Build history of the part. All positions in model axes, mm. Face numbers are marked on the shaded views. A direction names the side the tool comes from. Coordinates: 2 decimals unless noted, no trailing zeros. Loops run counter-clockwise (first coordinate to the right, second up) from the corner with the lowest first, then second, coordinate; pieces in that order, holes last.
(1) Slice it at A-A (z = 0). Give the cut face in (x, y) (3 decimals), and give its area (3 significant figures).
(2) Slice it at C-C (y = 9.25). Give the cut face in (x, z) (3 decimals).
(3) Two-plate mould, pull along X, no slides. Class the marked faces 3, 4 and 5: pulls with the +X half, pulls with the -X half, needs draft (parallel to the pull), parting line crosses it, or undercut.
(4) Wall check: L1, parallel to X at y = 11.75, z = 0 (3 decimals); L2, parallel to Y at x = 15.5, z = -11; L3, parallel to Z at x = 3, y = 4.25. Give the ranges that are in metal, low to high.
(5) Tool access for the marked faces 1 and 2: list every direction of +Z, -Z, +X, -X, +Y, -Y with a clear straight run to the whole face (end or side of a thin tool).
(6) Flat gauge pins, fed straight in: P1, Ø10, axis at y = 8, z = -2.5, coming from the -X side; P2, Ø1, axis at y = 17, z = -20, coming from the -X side; P3, Ø6, axis at x = -26.5, y = 11.5, coming from the +Z side; P4, Ø11.5, axis at x = 0, z = 0, coming from the -Y side. Where does each tip first touch, or does it go through?
(7) Slice it at B-B (x = 0). Give the cut face in (y, z) (3 decimals).
from build123d import *

# Parameters (mm, degrees)
SKETCH1_R           = 38.1
SKETCH1_R_2         = 9.525
BOSS_EXTRUDE1_DEPTH = 19.05
CHAMFER1_SIZE       = 2.54
SKETCH3_R           = 25.4
CUT_EXTRUDE2_DEPTH  = 6.35


with BuildPart() as part:
    # Sketch1 → Boss-Extrude1 (new body)
    with BuildSketch(Plane(origin=(0, 0, 0), x_dir=(1, 0, 0), z_dir=(0, 1, 0))):
        with Locations(Location((0, 0, 0), (0, 0, 90))):
            Circle(SKETCH1_R)
        with Locations(Location((0, 0, 0), (0, 0, 90))):
            Circle(SKETCH1_R_2, mode=Mode.SUBTRACT)
    extrude(amount=BOSS_EXTRUDE1_DEPTH)

    # Chamfer1
    chamfer1_edges = [part.edges().sort_by_distance(p)[0] for p in [
        (0, 0, 38.1),
        (0, 19.05, 38.1),
    ]]
    chamfer(chamfer1_edges, length=CHAMFER1_SIZE)

    # Sketch3 → Cut-Extrude2 (cut)
    with BuildSketch(Plane(origin=(0, 0, 0), x_dir=(-1, 0, 0), z_dir=(0, -1, 0))):
        with Locations(Location((0, 0, 0), (0, 0, 90))):
            Circle(SKETCH3_R)
    extrude(amount=-CUT_EXTRUDE2_DEPTH, mode=Mode.SUBTRACT)


solid = part.part
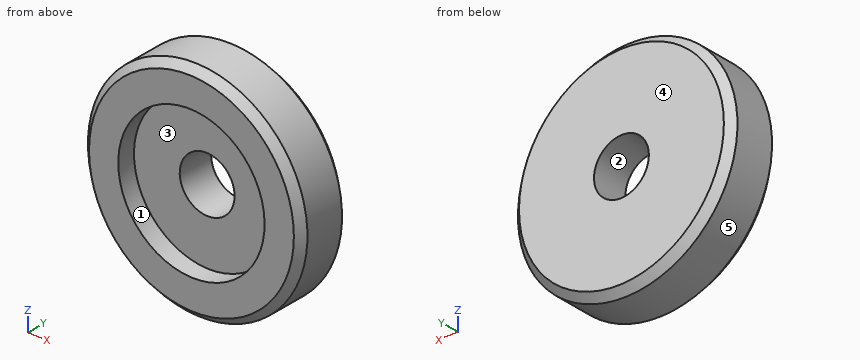
Response values:
1. outline: (-38.1, 2.54) - (-35.56, 0) - (-25.4, 0) - (-25.4, 6.35) - (-9.525, 6.35) - (-9.525, 19.05) - (-35.56, 19.05) - (-38.1, 16.51) - close; (9.525, 6.35) - (25.4, 6.35) - (25.4, 0) - (35.56, 0) - (38.1, 2.54) - (38.1, 16.51) - (35.56, 19.05) - (9.525, 19.05) - close
1. area: 874 mm2
2. outline: circle Ø76.2 at (0, 0); hole circle Ø19.05 at (0, 0)
3. face 3: undercut
3. face 4: needs draft
3. face 5: parting line crosses it
4. L1: x = -38.1 to -9.525, 9.525 to 38.1
4. L2: y = 6.35 to 19.05
4. L3: z = -37.98 to -25.22, 25.22 to 37.98
5. face 1: -Y
5. face 2: +Y, -Y
6. P1: stops at x = -38.1
6. P2: stops at x = -32.52
6. P3: stops at z = 29.99
6. P4: passes through
7. outline: (0, -35.56) - (2.54, -38.1) - (16.51, -38.1) - (19.05, -35.56) - (19.05, -9.525) - (6.35, -9.525) - (6.35, -25.4) - (0, -25.4) - close; (0, 25.4) - (6.35, 25.4) - (6.35, 9.525) - (19.05, 9.525) - (19.05, 35.56) - (16.51, 38.1) - (2.54, 38.1) - (0, 35.56) - close
